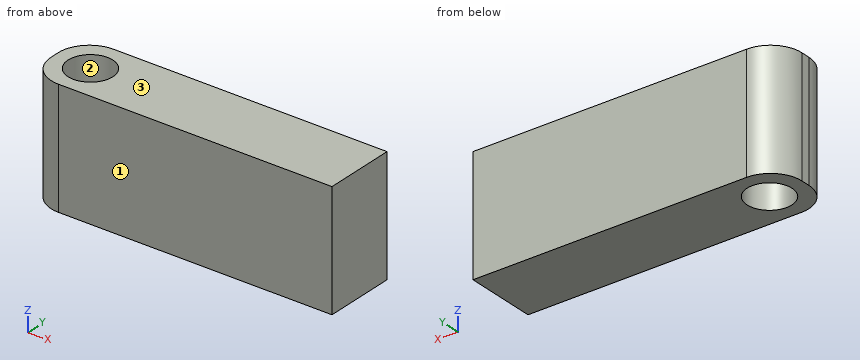
from build123d import *

# Parameters (mm, degrees)
SKETCH1_R           = 2.5
BOSS_EXTRUDE1_DEPTH = 6.5


with BuildPart() as part:
    # Sketch1 → Boss-Extrude1 (new body, symmetric)
    with BuildSketch(Plane.XY):
        with BuildLine():
            Line((-19.5, 34.428638458), (11, 34.428638458))
            Line((11, 34.428638458), (11, 26.428638458))
            Line((11, 26.428638458), (-19.5, 26.428638458))
            ThreePointArc((-19.5, 26.428638458), (-21.974873734, 27.453764724), (-23, 29.928638458))
            Line((-23, 29.928638458), (-23, 30.928638458))
            ThreePointArc((-23, 30.928638458), (-21.974873734, 33.403512192), (-19.5, 34.428638458))
        make_face()
        with Locations((-19, 30.428638458)):
            Circle(SKETCH1_R, mode=Mode.SUBTRACT)
    extrude(amount=BOSS_EXTRUDE1_DEPTH, both=True)


solid = part.part
The listing builds one solid part. Answer for the finished solid, in the listing's coordinates (mm). Face numbers are marked on the shaded views. Coordinates: 2 decimals unless noted, no trailing zeros. Order: outer loops, then holes, each group sorted by start corner. A loop starts at its lowest first (then second) coordinate and runs counter-clockwise, first axis right, second up.
Q1. Consider line 1 (Y direction, x = -19, z = -0.25); line 2 (X direction, y = 28.75, z = -2.25); line 3 (Y direction, x = -17, z = 3.75). Determine where each line is inside the solid, lowest interval first.
Q2. A cutting plane is placed at A-A, the plane x = -19. Write down the section's boundary in (y, z), and give its area (3 significant figures).
Q3. A cutting plane is placed at D-D, the plane y = 27.5. Write down the section's boundary in (x, z).
Q4. For a pull along Y with two mould halves and no side action, classify the marked faces 1, 2 and 3 as pulls with the +Y half, pulls with the -Y half, needs draft (parallel to the pull), parting line crosses it, or undercut.
Q5. A cutting plane is placed at B-B, the plane y = 32.25. Write down the section's boundary in (x, z), and give its area (3 significant figures).
Q6. A cutting plane is placed at C-C, the plane z = 4.25. Write down the section's boundary in (x, y), and give its area (3 significant figures).
Answers follow:
1. line 1: y = 26.43 to 27.93, 32.93 to 34.43
1. line 2: x = -22.8 to -20.85, -17.15 to 11
1. line 3: y = 26.43 to 28.93, 31.93 to 34.43
2. outline: (26.43, -6.5) - (27.93, -6.5) - (27.93, 6.5) - (26.43, 6.5) - close; (32.93, -6.5) - (34.43, -6.5) - (34.43, 6.5) - (32.93, 6.5) - close
2. area: 39.0 mm2
3. outline: (-22.02, -6.5) - (11, -6.5) - (11, 6.5) - (-22.02, 6.5) - close
4. face 1: pulls with the -Y half
4. face 2: undercut
4. face 3: needs draft
5. outline: (-22.74, -6.5) - (-20.71, -6.5) - (-20.71, 6.5) - (-22.74, 6.5) - close; (-17.29, -6.5) - (11, -6.5) - (11, 6.5) - (-17.29, 6.5) - close
5. area: 394 mm2
6. outline: (-23, 29.93) arc R3.5 ccw to (-19.5, 26.43) - (11, 26.43) - (11, 34.43) - (-19.5, 34.43) arc R3.5 ccw to (-23, 30.93) - close; hole circle Ø5 at (-19, 30.43)
6. area: 247 mm2
